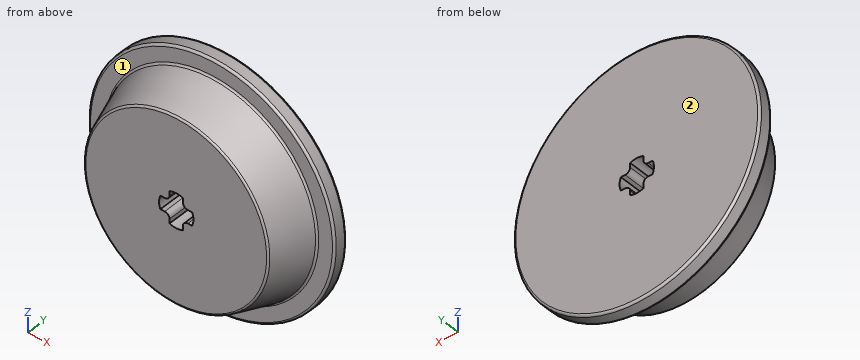
```python
from build123d import *

# Parameters (mm, degrees)
CUT_EXTRUDE1_DEPTH = 26.956426849
FILLET1_R          = 0.7
FILLET2_R          = 0.3


with BuildPart() as part:
    # Sketch2 → Revolve1 (revolve)
    with BuildSketch(Plane.XY, mode=Mode.PRIVATE) as revolve1_sk:
        Polygon((0, 0), (17.460470996, 0), (17.460470996, -2), (15, -2), (13.050481823, -8), (0, -8), align=None)
    revolve(revolve1_sk.sketch.rotate(Axis((0, 0, 0), (0, 1, 0)), 90), axis=Axis((0, 0, 0), (0, 1, 0)))

    # Sketch1 → Cut-Extrude1 (cut, through all)
    with BuildSketch(Plane(origin=(0, 0, 0), x_dir=(1, 0, 0), z_dir=(0, 1, 0))):
        with BuildLine():
            Line((-0.94, 0.94), (-2.25166605, 0.94))
            ThreePointArc((-2.25166605, 0.94), (-2.44, 0), (-2.25166605, -0.94))
            Line((-2.25166605, -0.94), (-0.94, -0.94))
            Line((-0.94, -0.94), (-0.94, -2.25166605))
            ThreePointArc((-0.94, -2.25166605), (0, -2.44), (0.94, -2.25166605))
            Line((0.94, -2.25166605), (0.94, -0.94))
            Line((0.94, -0.94), (2.25166605, -0.94))
            ThreePointArc((2.25166605, -0.94), (2.44, 0), (2.25166605, 0.94))
            Line((2.25166605, 0.94), (0.94, 0.94))
            Line((0.94, 0.94), (0.94, 2.25166605))
            ThreePointArc((0.94, 2.25166605), (0, 2.44), (-0.94, 2.25166605))
            Line((-0.94, 2.25166605), (-0.94, 0.94))
        make_face()
    extrude(amount=-CUT_EXTRUDE1_DEPTH, mode=Mode.SUBTRACT)

    # Fillet1
    fillet1_edges = [part.edges().sort_by_distance(p)[0] for p in [
        (-0.94, -4, -0.94),
        (0.94, -4, -0.94),
        (0.94, -4, 0.94),
        (-0.94, -4, 0.94),
    ]]
    fillet(fillet1_edges, radius=FILLET1_R)

    # Fillet2
    fillet2_edges = [part.edges().sort_by_distance(p)[0] for p in [
        (0, -8, 13.050481823),
        (0, -2, 15),
        (0, -2, 17.460470996),
        (0, 0, 17.460470996),
    ]]
    fillet(fillet2_edges, radius=FILLET2_R)


solid = part.part
```
Source: CAD feature listing. Evaluate the final solid. Frame: model axes, mm. Face numbers are marked on the shaded views. A direction names the side the tool comes from. Coordinates: 2 decimals unless noted, no trailing zeros. Write each loop counter-clockwise with the first axis right and the second up, starting at its lowest first coordinate (ties: lowest second). Pieces come first, ordered by that corner, then holes. Notation, with made-up numbers: M -2.5,-24.5 L 53.5,-24.5 A19 cw 53.5,-16.5 Z; hole C 88.5,-28.5 d2. An arc over 180 degrees is marked long. Answer as a JSON object with one key per item and string values.
1. Cut plane B-B on z = 0. Output: boundary loops of the cut face in (x, y).
Evaluation:
{"outline": "M -17.46,-1.7 A0.3 ccw -17.16,-2 L -15.22,-2 A0.3 cw -14.93,-2.21 L -13.12,-7.79 A0.3 ccw -12.83,-8 L -2.44,-8 L -2.44,0 L -17.16,0 A0.3 ccw -17.46,-0.3 Z; M 2.44,-8 L 12.83,-8 A0.3 ccw 13.12,-7.79 L 14.93,-2.21 A0.3 cw 15.22,-2 L 17.16,-2 A0.3 ccw 17.46,-1.7 L 17.46,-0.3 A0.3 ccw 17.16,0 L 2.44,0 Z"}
2. Access query for the marked faces 1 and 2. Directions: +Z, -Z, +X, -X, +Y, -Y. A direction counts if a zero-diameter tool reaches every point of the face in a straight line with its end or side. Return the directions, or none.
Evaluation:
{"face 1": "-Y", "face 2": "+Z, -Z, +X, -X, +Y"}
3. Contact query for flat-ended pins moving along their axis: P1, Ø0.7, axis at y = -3.5, z = 2, coming from the +X side; P2, Ø0.7, axis at y = -5.5, z = -2, coming from the -X side; P3, Ø0.5, axis at x = 2, y = -6, coming from the +Z side. Output: stop coordinate, or through.
Evaluation:
{"P1": "x = 14.5", "P2": "x = -13.84", "P3": "z = 13.64"}
4. Cut plane A-A on x = 0. Output: boundary loops of the cut face in (y, z).
Evaluation:
{"outline": "M -8,-12.83 A0.3 ccw -7.79,-13.12 L -2.21,-14.93 A0.3 cw -2,-15.22 L -2,-17.16 A0.3 ccw -1.7,-17.46 L -0.3,-17.46 A0.3 ccw 0,-17.16 L 0,-2.44 L -8,-2.44 Z; M -8,2.44 L 0,2.44 L 0,17.16 A0.3 ccw -0.3,17.46 L -1.7,17.46 A0.3 ccw -2,17.16 L -2,15.22 A0.3 cw -2.21,14.93 L -7.79,13.12 A0.3 ccw -8,12.83 Z"}
5. Cut plane C-C on y = -6.5. Output: boundary loops of the cut face in (x, z).
Evaluation:
{"outline": "C 0,0 d27.08; hole M -2.25,-0.94 L -1.64,-0.94 A0.7 cw -0.94,-1.64 L -0.94,-2.25 A2.44 ccw 0.94,-2.25 L 0.94,-1.64 A0.7 cw 1.64,-0.94 L 2.25,-0.94 A2.44 ccw 2.25,0.94 L 1.64,0.94 A0.7 cw 0.94,1.64 L 0.94,2.25 A2.44 ccw -0.94,2.25 L -0.94,1.64 A0.7 cw -1.64,0.94 L -2.25,0.94 A2.44 ccw Z"}
6. Ray query, L1, parallel to Y at x = 10, z = -14; L2, parallel to Z at x = -1.5, y = -2.25; L3, parallel to X at y = -6, z = -1.5. Return the intervals inside material, ascending.
Evaluation:
{"L1": "-2 to 0", "L2": "-14.84 to -0.95, 0.95 to 14.84", "L3": "-13.62 to -0.95, 0.95 to 13.62"}
